from build123d import *

# Parameters (mm, degrees)
F1_DEPTH = 10.16


with BuildPart() as f1:
    # F0 (on Top) → F1 (new body)
    with BuildSketch(Plane.XY):
        Polygon((44.45, 0), (31.75, 0), (31.75, -10.16), (10.16, -10.16), (10.16, -31.75), (0, -31.75), (0, -44.45), (10.16, -44.45), (10.16, -57.15), (0, -57.15), (0, -69.85), (10.16, -69.85), (10.16, -82.55), (0, -82.55), (0, -95.25), (10.16, -95.25), (10.16, -107.95), (0, -107.95), (0, -120.65), (10.16, -120.65), (10.16, -133.35), (0, -133.35), (0, -146.05), (10.16, -146.05), (10.16, -167.64), (31.75, -167.64), (31.75, -177.8), (44.45, -177.8), (44.45, -167.64), (57.15, -167.64), (57.15, -177.8), (69.85, -177.8), (69.85, -167.64), (82.55, -167.64), (82.55, -177.8), (95.25, -177.8), (95.25, -167.64), (107.95, -167.64), (107.95, -177.8), (120.65, -177.8), (120.65, -167.64), (133.35, -167.64), (133.35, -177.8), (146.05, -177.8), (146.05, -167.64), (158.75, -167.64), (158.75, -177.8), (171.45, -177.8), (171.45, -167.64), (184.15, -167.64), (184.15, -177.8), (196.85, -177.8), (196.85, -167.64), (209.55, -167.64), (209.55, -177.8), (222.25, -177.8), (222.25, -167.64), (243.84, -167.64), (243.84, -146.05), (254, -146.05), (254, -133.35), (243.84, -133.35), (243.84, -120.65), (254, -120.65), (254, -107.95), (243.84, -107.95), (243.84, -95.25), (254, -95.25), (254, -82.55), (243.84, -82.55), (243.84, -69.85), (254, -69.85), (254, -57.15), (243.84, -57.15), (243.84, -44.45), (254, -44.45), (254, -31.75), (243.84, -31.75), (243.84, -10.16), (222.25, -10.16), (222.25, 0), (209.55, 0), (209.55, -10.16), (196.85, -10.16), (196.85, 0), (184.15, 0), (184.15, -10.16), (171.45, -10.16), (171.45, 0), (158.75, 0), (158.75, -10.16), (146.05, -10.16), (146.05, 0), (133.35, 0), (133.35, -10.16), (120.65, -10.16), (120.65, 0), (107.95, 0), (107.95, -10.16), (95.25, -10.16), (95.25, 0), (82.55, 0), (82.55, -10.16), (69.85, -10.16), (69.85, 0), (57.15, 0), (57.15, -10.16), (44.45, -10.16), align=None)
    extrude(amount=F1_DEPTH)


solid = f1.part
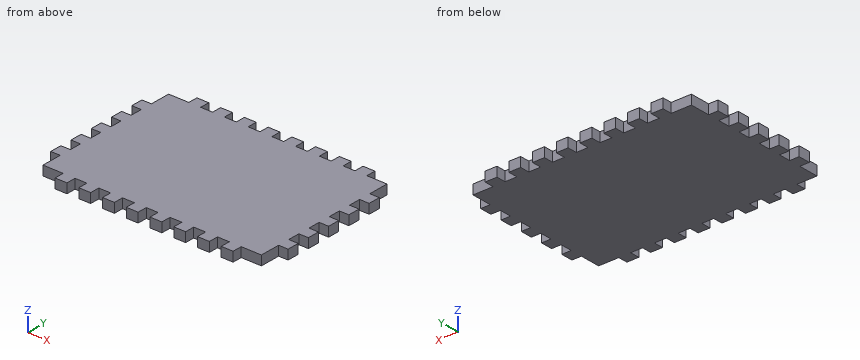
The listing builds one solid part. Answer for the finished solid, in the listing's coordinates (mm). Give positions to 0.01 mm unless a question says otherwise; leave off trailing zeros. Loops run counter-clockwise (first coordinate to the right, second up) from the corner with the lowest first, then second, coordinate; pieces in that order, holes last. Notation, with made-up numbers: (20, 18.5) - (40, 18.5) arc R31 ccw to (40, 51.5) - close; hole circle Ø11 at (81, 85). An arc over 180 degrees is marked (long way). Answer as a JSON object with one key per item and string values.
1. Find the intervals of material crossed by L1, parallel to Y at x = 71, z = 6.75; L2, parallel to X at y = -157, z = 5, in increasing order. Write a range as [from, to].
Determined:
{"L1": "[-167.64, -10.16]", "L2": "[10.16, 243.84]"}
2. Flat-ended cylindrical pins translate along their axes: pin 1 Ø3 at (x, z) = (2.5, 6.5) entering from -Y; pin 2 Ø3 at (y, z) = (-6.5, 6.5) entering from +X; pin 3 Ø5 at (y, z) = (-78.5, 3.5) entering from -X. Find the tip coordinate at first contact, or state that the pin passes through.
Determined:
{"pin 1": "y = -146.05", "pin 2": "x = 222.25", "pin 3": "x = 10.16"}
3. A cutting plane is placed at A-A (x = 176). Write down the section's boundary in (y, z), then the cut area to 3 significant figures.
Determined:
{"outline": "(-167.64, 0) - (-10.16, 0) - (-10.16, 10.16) - (-167.64, 10.16) - close", "area": "1,600 mm²"}
4. A cutting plane is placed at B-B (y = -27). Write down the section's boundary in (x, z), then the cut area to 3 significant figures.
Determined:
{"outline": "(10.16, 0) - (243.84, 0) - (243.84, 10.16) - (10.16, 10.16) - close", "area": "2,370 mm²"}
